CAD build for the part. Positions are in the model's coordinates, mm. Round coordinates to 2 decimals unless told otherwise and drop trailing zeros. Write each loop counter-clockwise with the first axis right and the second up, starting at its lowest first coordinate (ties: lowest second). Pieces come first, ordered by that corner, then holes. Notation, with made-up numbers: (-1, 39) - (31, 39) arc R20 cw to (31, 47) - close; hole circle Ø11 at (76.25, 38.5). An arc over 180 degrees is marked (long way). Put each result on its own line as item: value. Start each with the question number.
Item 1: Cut at A-A (x = 0). Give the cut face in (y, z) (3 decimals), and give its area (3 significant figures).
Item 2: Pin check, flat tips, straight feed: pin 1 Ø3 at (x, z) = (8, 6.5) entering from +Y; pin 2 Ø1 at (y, z) = (-23, 7.5) entering from +X; pin 3 Ø1.5 at (y, z) = (-10.5, 3) entering from +X. Stop position of each tip, or through.
Item 3: Mould opens along Y. For faces 1 (the cylindrical face through (-5.5, -24.9, 1.1)), 2 (the cylindrical face through (13.797, -26.526, 4.93)), 3 (the cylindrical face through (-5.5, -24.9, 9)), 4 (the flat face through (22, 13.4, 0)) say: released by +Y, released by -Y, zero draft, split by the parting line, or undercut.
Item 4: Cut at B-B (z = 3.75). Give the cut face in (x, y).
Item 5: Drill centre lines: line 1 (Y direction, x = 0, z = 8.4); line 2 (Y direction, x = 16, z = 8.75); line 3 (X direction, y = -15.5, z = 6.5). Where is each one in solid material? Low to high. Write a range as from..to.
```python
from build123d import *

# Parameters (mm, degrees)
SKETCH1_R           = 29.9
BOSS_EXTRUDE1_DEPTH = 10
CUT_EXTRUDE1_REACH  = 12
SKETCH2_R           = 25.5
SKETCH3_R           = 3.275


with BuildPart() as part:
    # Sketch1 → Boss-Extrude1 (new body)
    with BuildSketch(Plane.XY):
        Circle(SKETCH1_R)
    extrude(amount=BOSS_EXTRUDE1_DEPTH)

    # Sketch2 → Cut-Extrude1 (cut, up to next)
    with BuildSketch(Plane.XY.offset(10), mode=Mode.PRIVATE) as cut_extrude1_sk1:
        Circle(SKETCH2_R)
    cut_extrude1_tool1 = extrude(cut_extrude1_sk1.sketch, amount=-CUT_EXTRUDE1_REACH, mode=Mode.PRIVATE) & part.part
    add(cut_extrude1_tool1.solids().sort_by_distance((0, 0, 10))[0], mode=Mode.SUBTRACT)

    # Sketch3 → Cut-Revolve2 (revolve, cut)
    with BuildSketch(Plane(origin=(0, 0, 0), x_dir=(1, 0, 0), z_dir=(0, 1, 0))):
        with Locations((-24, -5)):
            Circle(SKETCH3_R)
    revolve(axis=Axis((0, 0, -18.462767292), (0, 0, 1)), mode=Mode.SUBTRACT)


solid = part.part
```
Output values:
1. outline: (-29.9, 0) - (-25.5, 0) - (-25.5, 2.089) arc R3.275 cw to (-25.5, 7.911) - (-25.5, 10) - (-29.9, 10) - close; (25.5, 0) - (29.9, 0) - (29.9, 10) - (25.5, 10) - (25.5, 7.911) arc R3.275 cw to (25.5, 2.089) - close
1. area: 73.2 mm2
2. pin 1: y = 29.18
2. pin 2: x = 19.69
2. pin 3: x = 28.27
3. face 1: undercut
3. face 2: split by the parting line
3. face 3: undercut
3. face 4: zero draft
4. outline: circle Ø59.8 at (0, 0); hole circle Ø54.05 at (0, 0)
5. line 1: -29.9..-25.5, 25.5..29.9
5. line 2: -25.26..-19.86, 19.86..25.26
5. line 3: -25.57..-22, 22..25.57
